Solid Edge part; units mm, degrees
sketch "Sketch1" plane through (0, 0, 0) normal (0, 0, 1) x (1, 0, 0)
  arc A0 (-2.1, 0) -> (-1.311, 2.3853) centre (1.9, 0) cw
  line L0 (-1.311, 2.3853) -> (0, 2.5)
  line L1 (0, 2.5) -> (0, 1.212)
  arc A1 (0, 1.212) -> (0.1, 1.112) centre (0.1, 1.212) ccw
  line L2 (0.1, 1.112) -> (0.9, 1.25)
  line L3 (0.9, 1.25) -> (5.8048, 1.25)
  line L4 (5.8048, 1.25) -> (6, 0.974)
  line L5 (6, 0.974) -> (6, 0)
  line L6 (6, 0) -> (-2.1, 0)
revolve "RevolvedProtrusion1" add sketch "Sketch1" angle 360 about axis through (6, 0, 0) along (-1, 0, 0)
sketch "Sketch2" plane through (-2.1, 0, 0) normal (1, 0, 0) x (0, 1, 0)
  line L0 (0.3375, 1.35) -> (-0.3375, 1.35)
  line L1 (-0.3375, 1.35) -> (-0.2666, 0.54)
  line L2 (-0.2666, 0.54) -> (-0.3375, 0.3375)
  line L3 (-0.3375, 0.3375) -> (-0.54, 0.2666)
  line L4 (-0.54, 0.2666) -> (-1.35, 0.3375)
  line L5 (-1.35, 0.3375) -> (-1.35, -0.3375)
  line L6 (-1.35, -0.3375) -> (-0.54, -0.2666)
  line L7 (-0.54, -0.2666) -> (-0.3375, -0.3375)
  line L8 (-0.3375, -0.3375) -> (-0.2666, -0.54)
  line L9 (-0.2666, -0.54) -> (-0.3375, -1.35)
  line L10 (-0.3375, -1.35) -> (0.3375, -1.35)
  line L11 (0.3375, -1.35) -> (0.2666, -0.54)
  line L12 (0.2666, -0.54) -> (0.3375, -0.3375)
  line L13 (0.3375, -0.3375) -> (0.54, -0.2666)
  line L14 (0.54, -0.2666) -> (1.35, -0.3375)
  line L15 (1.35, -0.3375) -> (1.35, 0.3375)
  line L16 (1.35, 0.3375) -> (0.54, 0.2666)
  line L17 (0.54, 0.2666) -> (0.3375, 0.3375)
  line L18 (0.3375, 0.3375) -> (0.2666, 0.54)
  line L19 (0.2666, 0.54) -> (0.3375, 1.35)
extrude "ExtrudedCutout_1" cut sketch "Sketch2" along normal blind 1.05
properties part number "SFS FN 405 146084 Flachkopfschraube ISO 7045 Stahl 4.8 verzinkt blau M2.5x6-H"
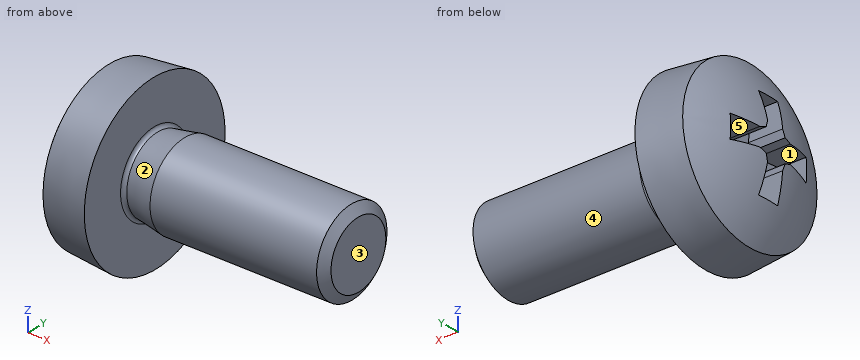
CAD build for the part. Positions are in the model's coordinates, mm. Face numbers are marked on the shaded views. A direction names the side the tool comes from. Coordinates: 2 decimals unless noted, no trailing zeros. Write each loop counter-clockwise with the first axis right and the second up, starting at its lowest first coordinate (ties: lowest second). Pieces come first, ordered by that corner, then holes.
(1) Two-plate mould, pull along Y, no slides. Class the marked faces 1, 2 and 3: +Y half, -Y half, draft (parallel to the pull), parting line (faces both ways), or undercut.
(2) Cut at A-A, the plane z = 0. List the corners of the cut face in (x, y), and give its area (3 significant figures).
(3) Drill centre lines: probe 1 along Z at (x, y) = (1, 0); probe 2 along X at (y, z) = (0.25, 0.35); probe 3 along Y at (x, z) = (-1.5, 1.25). Where is each one in solid material? Low to high.
(4) Flat gauge pins, fed straight in: pin 1 (2.5 mm diameter, centred on y = 0, z = -1, fed in from +X); pin 2 (0.5 mm diameter, centred on x = -1.5, y = 0, fed in from -Z); pin 3 (3 mm diameter, centred on x = 3.5, z = 2, fed in from -Y); pin 4 (0.7 mm diameter, centred on x = -1.5, y = 0, fed in from +Z). Where does each tip first touch, or does it go through?
(5) 3-axis set-ups, long thin cutter, end or side, ignore diameter. For the marked faces 4 and 5: which of +Z, -Z, +X, -X, +Y, -Y reach the whole face in a straight line?
(6) Cut at C-C, the plane x = 3.75. List the corners of the cut face in (y, z), and give its area (3 significant figures).
(7) Cut at D-D, the plane x = 0.25. List the corners of the cut face in (y, z).
Geometry says:
1. face 1: undercut
1. face 2: parting line
1. face 3: draft
2. outline: (-1.87, -1.35) arc R4 ccw to (-1.31, -2.39) - (0, -2.5) - (0, -1.21) arc R0.1 cw to (0.1, -1.11) - (0.9, -1.25) - (5.8, -1.25) - (6, -0.97) - (6, 0.97) - (5.8, 1.25) - (0.9, 1.25) - (0.1, 1.11) arc R0.1 cw to (0, 1.21) - (0, 2.5) - (-1.31, 2.39) arc R4 ccw to (-1.87, 1.35) - (-1.05, 1.35) - (-1.05, -1.35) - close
2. area: 21.2 mm2
3. probe 1: z = -1.25 to 1.25
3. probe 2: x = -1.05 to 6
3. probe 3: y = -1.7 to -0.33, 0.33 to 1.7
4. pin 1: stops at x = 6
4. pin 2: stops at z = -2.39
4. pin 3: stops at y = -1.15
4. pin 4: stops at z = 2.4
5. face 4: +X
5. face 5: -X
6. outline: circle Ø2.5 at (0, 0)
6. area: 4.91 mm2
7. outline: circle Ø2.28 at (0, 0)
